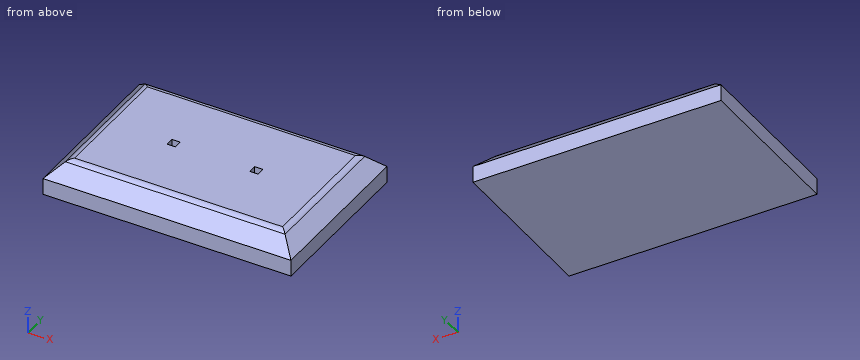
```python
from build123d import *

# Parameters (mm, degrees)
F0_W     = 150
F0_H     = 100
F1_DEPTH = 20
F2_SIZE  = 10
F3_W     = 2.5
F3_H     = 2.5
F4_DEPTH = 10
F5_R     = 5


with BuildPart() as f1:
    # F0 (on Top) → F1 (new body)
    with BuildSketch(Plane.XY):
        with Locations((9.132270515, -50)):
            Rectangle(F0_W, F0_H)
    extrude(amount=F1_DEPTH)

    # F2
    f2_edges = [f1.edges().sort_by_distance(p)[0] for p in [
        (9.132271, -100, 20),
        (-65.867729, -50, 20),
        (9.132271, 0, 20),
        (84.132271, -50, 20),
    ]]
    chamfer(f2_edges, length=F2_SIZE)

    # F3 (on face) → F4 (cut)
    with BuildSketch(Plane.XY.offset(20)):
        Polygon((-18.367729485, -47.5), (-18.367729485, -50), (-15.867729485, -50), (-13.367729485, -50), (-13.367729485, -47.5), (-15.867729485, -47.5), align=None)
        Polygon((-15.867729485, -50), (-18.367729485, -50), (-18.367729485, -52.5), (-13.367729485, -52.5), (-13.367729485, -50), align=None)
        with Locations((32.882270515, -48.75)):
            Rectangle(F3_W, F3_H)
        Polygon((34.132270515, -50), (31.632270515, -50), (31.632270515, -52.5), (36.632270515, -52.5), (36.632270515, -50), align=None)
        with Locations((35.382270515, -48.75)):
            Rectangle(F3_W, F3_H)
    extrude(amount=-F4_DEPTH, mode=Mode.SUBTRACT)

    # F5
    f5_edges = [f1.edges().sort_by_distance(p)[0] for p in [
        (9.132271, -90, 20),
        (-55.867729, -50, 20),
        (74.132271, -50, 20),
        (9.132271, -10, 20),
    ]]
    fillet(f5_edges, radius=F5_R)


solid = f1.part
```
Can you work these out from the model? Positions are in its coordinate system, mm. Coordinates: 2 decimals unless noted, no trailing zeros. Write each loop counter-clockwise with the first axis right and the second up, starting at its lowest first coordinate (ties: lowest second). Pieces come first, ordered by that corner, then holes. Notation, with made-up numbers: M -14,63 L 21,63 A28 cw 21,88 Z; hole C 63.5,15 d10. An arc over 180 degrees is marked long. Write item = value, one per line. Start each with the question number.
Q1. If we section it at A-A, the plane y = -20.5: Write out the boundary of the cut face in (x, z).
Q2. If we section it at D-D, the plane y = -49: Write out the boundary of the cut face in (x, z).
Q3. I'm going to push flat-ended pins straight in: pin 1 (2.5 mm diameter, centred on y = -50.5, z = 12.5, fed in from -X); pin 2 (5.5 mm diameter, centred on x = -16.5, z = 16.5, fed in from +Y); pin 3 (5.5 mm diameter, centred on x = 35, z = 12.5, fed in from -Y); pin 4 (5.5 mm diameter, centred on y = -49, z = 16, fed in from +X). Where does each tip first touch, or does it pass through?
Q4. If we section it at B-B, the plane x = 8: Write out the boundary of the cut face in (y, z).
Q5. If we section it at C-C, the plane z = 15: Write out the boundary of the cut face in (x, y).
Q6. If I drill on L1, parallel to Z at x = -54, y = -55; L2, parallel to Y at x = 19.5, z = 18.5; L3, parallel to X at y = -51, z = 10.25, over which ranges is the centre line in solid material (lowest first)? Write a range as [from, to].
Check sheet entries:
q1.outline = M -65.87,0 L 84.13,0 L 84.13,10 L 75.6,18.54 A5 ccw 72.06,20 L -53.8,20 A5 ccw -57.33,18.54 L -65.87,10 Z
q2.outline = M -65.87,0 L 84.13,0 L 84.13,10 L 75.6,18.54 A5 ccw 72.06,20 L 36.63,20 L 36.63,10 L 31.63,10 L 31.63,20 L -13.37,20 L -13.37,10 L -18.37,10 L -18.37,20 L -53.8,20 A5 ccw -57.33,18.54 L -65.87,10 Z
q3.pin_1 = -64.62
q3.pin_2 = -3.75
q3.pin_3 = -100
q3.pin_4 = 80.88
q4.outline = M -100,0 L 0,0 L 0,10 L -8.54,18.54 A5 ccw -12.07,20 L -87.93,20 A5 ccw -91.46,18.54 L -100,10 Z
q5.outline = M -60.87,-95 L 79.13,-95 L 79.13,-5 L -60.87,-5 Z; hole M -18.37,-52.5 L -13.37,-52.5 L -13.37,-47.5 L -18.37,-47.5 Z; hole M 31.63,-52.5 L 36.63,-52.5 L 36.63,-47.5 L 31.63,-47.5 Z
q6.L1 = [0, 20]
q6.L2 = [-91.5, -8.5]
q6.L3 = [-65.62, -18.37], [-13.37, 31.63], [36.63, 83.88]
